Geometry check sheet. Reference: the model listing, model coordinates, mm. A direction names the side the tool comes from. Round coordinates to 2 decimals unless told otherwise and drop trailing zeros.
Item 1: Cross-section at A-A (y = 3). State how many separate pieces and enclosed holes the cut face has, then the cut area to 3 significant figures.
Item 2: Access from +Z, -Z, +X, -X, +Y, -Y to the whole of each face (thin tool, end or side, straight path). Record for faces 3 (the face through (0, 2.5, 0)), 4 (the face through (0, 0, 9)).
Item 3: Scan lines: probe 1 along X at (y, z) = (5, 0) (3 decimals); probe 2 along X at (y, z) = (4, 0) (3 decimals); probe 3 along Z at (x, y) = (4, 2.5). Record each from-to range of solid material in increasing order.
Item 4: Draft check along X on faces 1 (the face through (0, 7.5, 0)), 2 (the face through (-6.76, 3.45, 1.5)). Enter one of: pulls with the +X half, pulls with the -X half, needs draft (parallel to the pull), parting line crosses it, or undercut.
Item 5: Depth check by flat-ended pin: P1, Ø3, axis at y = 5, z = -0.5, coming from the +X side; P2, Ø3, axis at x = -13, y = 1, coming from the +Z side; P3, Ø8, axis at x = -15, z = 14, coming from the +Y side. Enter the tip coordinate at first touch or a pass-through.
from build123d import *

# Parameters (mm, degrees)
SKETCH1_R           = 20
BOSS_EXTRUDE1_DEPTH = 7.5
FILLET1_R           = 20
SKETCH2_R           = 6.925
CUT_EXTRUDE1_DEPTH  = 7
SKETCH3_R           = 4.558249482
CUT_EXTRUDE2_DEPTH  = 2.5


with BuildPart() as part:
    # Sketch1 → Boss-Extrude1 (new body)
    with BuildSketch(Plane(origin=(0, 0, 0), x_dir=(1, 0, 0), z_dir=(0, 1, 0))):
        with Locations(Location((0, 0, 0), (0, 0, 270))):
            Circle(SKETCH1_R)
    extrude(amount=BOSS_EXTRUDE1_DEPTH)

    # Fillet1
    # the kernel refuses this fillet: 20 mm, written as the material it takes off along each edge
    with BuildSketch(Plane(origin=(0, 7.5, 0), x_dir=(0, 0, 1), z_dir=(-1, 0, 0))) as fillet1_piece_1:
        with BuildLine():
            CenterArc((4.387505004, -20), FILLET1_R, 38.682187453, 51.317812547)
            Line((4.387505004, 0), (4.387505004, 0.4))
            Line((4.387505004, 0.4), (20, 0.4))
            Line((20, 0.4), (20.4, 0))
            ThreePointArc((20.4, 0), (20.4, -3.75), (20.3122499, -7.25))
            Line((20.3122499, -7.25), (20, -7.5))
        make_face()
    revolve(axis=Axis((0, 7.5, 0), (0, 1, 0)), mode=Mode.SUBTRACT)

    # Sketch2 → Cut-Extrude1 (cut)
    with BuildSketch(Plane.XZ):
        with Locations(Location((0, 0, 0), (0, 0, 270))):
            Circle(SKETCH2_R)
        Polygon((3.1, -1.789785834), (3.1, 1.789785834), (0, 3.579571669), (-3.1, 1.789785834), (-3.1, -1.789785834), (0, -3.579571669), align=None, mode=Mode.SUBTRACT)
    extrude(amount=-CUT_EXTRUDE1_DEPTH, mode=Mode.SUBTRACT)

    # Sketch3 → Cut-Extrude2 (cut)
    with BuildSketch(Plane.XZ):
        Circle(SKETCH3_R)
    extrude(amount=-CUT_EXTRUDE2_DEPTH, mode=Mode.SUBTRACT)


solid = part.part
Resolved:
1. separate pieces: 2
1. enclosed holes: 1
1. area: 793 mm2
2. face 3: -Y
2. face 4: +Z, -Z, +X, -X, -Y
3. probe 1: x = -14.07 to -6.925, -3.1 to 3.1, 6.925 to 14.07
3. probe 2: x = -15.69 to -6.925, -3.1 to 3.1, 6.925 to 15.69
3. probe 3: z = -17.16 to -5.65, 5.65 to 17.16
4. face 1: needs draft
4. face 2: undercut
5. P1: stops at x = 16.38
5. P2: stops at z = 16.09
5. P3: stops at y = 3.4
